from build123d import *

# Parameters (mm, degrees)
SKETCH_1_R      = 1.5
EXTRUDE_1_DEPTH = 5
EXTRUDE_2_DEPTH = 9
CHAMFER_1_SIZE  = 0.2


with BuildPart() as part:
    # Эскиз1 → Бобышка-Вытянуть1 (new body)
    with BuildSketch(Plane.XY):
        Circle(SKETCH_1_R)
    extrude(amount=EXTRUDE_1_DEPTH)

    # Эскиз2 → Бобышка-Вытянуть2 (add)
    with BuildSketch(Plane.XY.offset(5)):
        with BuildLine():
            Line((1.1, 1.019803903), (1.1, -1.019803903))
            ThreePointArc((1.1, -1.019803903), (-1.5, 0), (1.1, 1.019803903))
        make_face()
    extrude(amount=EXTRUDE_2_DEPTH)

    # Фаска1
    chamfer_1_edges = [part.edges().sort_by_distance(p)[0] for p in [
        (-1.5, 0, 14),
    ]]
    chamfer(chamfer_1_edges, length=CHAMFER_1_SIZE)


solid = part.part
Source: CAD feature listing. Evaluate the final solid. Frame: model axes, mm. A direction names the side the tool comes from. Give positions to 0.01 mm unless a question says otherwise; leave off trailing zeros. Write each loop counter-clockwise with the first axis right and the second up, starting at its lowest first coordinate (ties: lowest second). Pieces come first, ordered by that corner, then holes. Notation, with made-up numbers: (42.25, -29) -> (81.25, -29) arc R24 cw to (81.25, -6) -> close; hole circle Ø5 at (86, 34). An arc over 180 degrees is marked (long way). Return JSON: item names as keys, results as strings. Group by question number.
1. Access query for faces 1 (the face through (1.1, 0, 9)), 2 (the face through (0, 0, 0)). Directions: +Z, -Z, +X, -X, +Y, -Y. A direction counts if a zero-diameter tool reaches every point of the face in a straight line with its end or side. Return the directions, or none.
2. Section B-B, the plane z = 4.5. Output: boundary loops of the cut face in (x, y).
3. Section A-A, the plane z = 13.25. Output: boundary loops of the cut face in (x, y).
4. Material intervals for line 1 (Y direction, x = -0.1, z = 8.25); line 2 (X direction, y = -0.75, z = 3.75); line 3 (X direction, y = -1.1, z = 7.5), sorted ascending. Write a range as from..to.
Determined:
{
 "1": {"face 1": "+Z, +X, +Y, -Y", "face 2": "-Z, +X, -X, +Y, -Y"},
 "2": {"outline": "circle Ø3 at (0, 0)"},
 "3": {"outline": "(1.1, -1.02) -> (1.1, 1.02) arc R1.5 ccw (long way) to start"},
 "4": {"line 1": "y = -1.5..1.5", "line 2": "x = -1.3..1.3", "line 3": "x = -1.02..1.02"}
}
